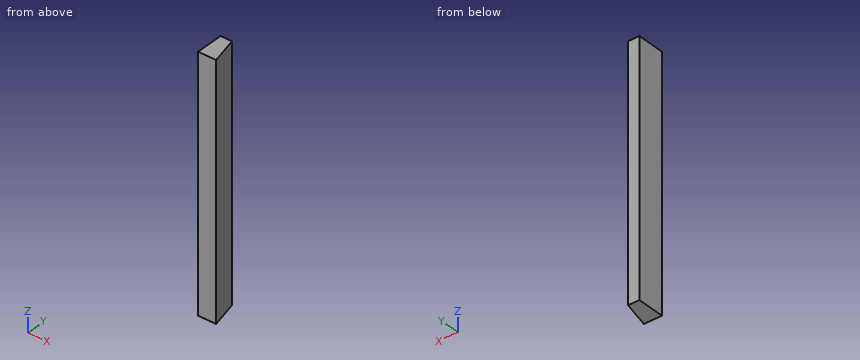
Autodesk Inventor part; units mm, degrees
ref_plane "Work Plane1" through (-812.8, 0, -698.5) normal (0, 0, -1) x (0, 1, 0)
ref_plane "YZ Plane" through (0, 0, 0) normal (1, 0, 0) x (0, 1, 0)
ref_plane "XZ Plane" through (0, 0, 0) normal (0, 1, 0) x (-1, 0, 0)
sketch "Sketch1" plane through (0, 0, 0) normal (0, 0, 1) x (1, 0, 0)
  line L0 (-812.8, -3.937) -> (0, -3.937)
  line L1 (0, 73.787) -> (-812.8, 73.787)
  line L2 (-813.562, 73.533) -> (-813.562, -3.175)
  line L3 (-762.762, -3.937) -> (-762.762, -7.112)
  line L4 (-781.812, 77.47) -> (-781.812, 74.295)
  line L5 (-762.762, -3.937) -> (-813.562, -3.937)
  line L6 (-813.562, -3.937) -> (-813.562, 73.787)
  line L7 (-813.562, 73.787) -> (-781.6883, 73.787)
  line L8 (-781.6883, 73.787) -> (-762.762, -3.937)
  point P0 (0, 0)
ref_plane "Work Plane1" through (-812.8, 0, -698.5) normal (0, 0, -1) x (0, 1, 0)
extrude "Extrusion1" add sketch "Sketch1" against normal up to surface (698.5 mm away)
properties part number "RearBumperFill"
Geometry check sheet. Reference: the model listing, model coordinates, mm. Coordinates: 2 decimals unless noted, no trailing zeros. Order: outer loops, then holes, each group sorted by start corner. A loop starts at its lowest first (then second) coordinate and runs counter-clockwise, first axis right, second up.
Q1. Thickness scan on probe 1 along X at (y, z) = (36.5, -594); probe 2 along X at (y, z) = (40, -336). Record the ranges inside material, lowest first.
Reply:
probe 1: x = -813.56 to -772.61
probe 2: x = -813.56 to -773.46
Q2. Sectioned sample at A-A on z = -414. Record the cut outline in (x, y).
Reply:
outline: (-813.56, -3.94) - (-762.76, -3.94) - (-781.69, 73.79) - (-813.56, 73.79) - close
Q3. Sectioned sample at B-B on y = 36. Record the cut outline in (x, z).
Reply:
outline: (-813.56, -698.5) - (-772.49, -698.5) - (-772.49, 0) - (-813.56, 0) - close
Q4. Depth check by flat-ended pin: pin 1 Ø5 at (x, y) = (-805, 8.5) entering from +Z; pin 2 Ø6 at (y, z) = (40.5, -377) entering from +X; pin 3 Ø6 at (y, z) = (63, -380.5) entering from +X. Enter the tip coordinate at first touch or a pass-through.
Reply:
pin 1: stops at z = 0
pin 2: stops at x = -772.85
pin 3: stops at x = -778.33
